For this review, take the finished solid that the model builds, in its own axes (mm). Face numbers are marked on the shaded views. A direction names the side the tool comes from. Round coordinates to 2 decimals unless told otherwise and drop trailing zeros. Order: outer loops, then holes, each group sorted by start corner. A loop starts at its lowest first (then second) coordinate and runs counter-clockwise, first axis right, second up. Notation, with made-up numbers: M 64.5,-39.5 L 92.5,-39.5 A27 cw 92.5,-23.5 Z; hole C -12.75,86 d4. An arc over 180 degrees is marked long. Answer as a JSON object with one key per item and string values.
from build123d import *

# Parameters (mm, degrees)
F0_R     = 19.2
F1_DEPTH = 10
F2_R     = 17
F3_DEPTH = 8
F4_R     = 5.25
F4_R_2   = 3.35
F5_DEPTH = 10
F7_DEPTH = 9
F8_W     = 1
F8_H     = 1
F9_DEPTH = 10


with BuildPart() as f1:
    # F0 (on Top) → F1 (new body)
    with BuildSketch(Plane.XY):
        Circle(F0_R)
    extrude(amount=F1_DEPTH)

    # F2 (on Top) → F3 (cut)
    with BuildSketch(Plane.XY):
        Circle(F2_R)
    extrude(amount=F3_DEPTH, mode=Mode.SUBTRACT)

    # F4 (on Top) → F5 (join)
    with BuildSketch(Plane.XY):
        Circle(F4_R)
        Circle(F4_R_2, mode=Mode.SUBTRACT)
    extrude(amount=F5_DEPTH)

    # F6 (on Top) → F7 (join)
    with BuildSketch(Plane.XY):
        with BuildLine():
            Line((4.017093, -1.060893), (-3.993784, -1.060893))
            ThreePointArc((-3.993784, -1.060893), (0.011655, -3.969964), (4.017093, -1.060893))
        make_face()
    extrude(amount=F7_DEPTH)

    # F8 (on Top) → F9 (join)
    with BuildSketch(Plane.XY):
        with Locations((0, -19.229485)):
            Rectangle(F8_W, F8_H)
    extrude(amount=F9_DEPTH)


solid = f1.part
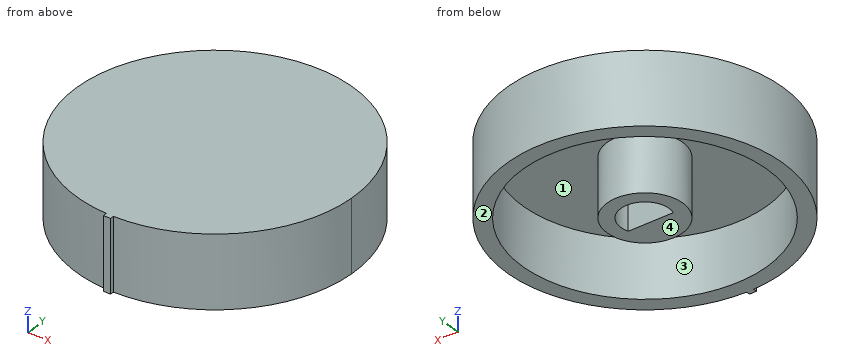
1) For L1, parallel to Y at x = 0, z = 5.25; L2, parallel to X at y = -2, z = 4.5; L3, parallel to X at y = 1, z = 2.5, list the stretches that pass through material, from the lowest coordinate up.
Geometry check:
{"L1": "y = -19.73 to -17, -5.25 to -1.06, 3.35 to 5.25, 17 to 19.2", "L2": "x = -19.1 to -16.88, -4.85 to 4.85, 16.88 to 19.1", "L3": "x = -19.17 to -16.97, -5.15 to -3.2, 3.2 to 5.15, 16.97 to 19.17"}
2) Add section A-A on z = 4.5. State the section outline as (x, y) points.
Geometry check:
{"outline": "C 0,0 d10.5; M -0.5,-19.73 L 0.5,-19.73 L 0.5,-19.19 A19.2 ccw long -0.5,-19.19 Z; hole C 0,0 d34; hole M -3.18,-1.06 L 3.18,-1.06 A3.35 ccw long Z"}
3) Mouldability with a two-part tool opening along X and no side actions: class the marked faces 1 and 2 as +X half, -X half, draft (parallel to the pull), parting line (faces both ways), or undercut.
Geometry check:
{"face 1": "undercut", "face 2": "draft"}
4) Add section B-B on x = 0. State the section outline as (y, z) points, and give its area (3 significant figures).
Geometry check:
{"outline": "M -19.73,0 L -17,0 L -17,8 L -5.25,8 L -5.25,0 L -1.06,0 L -1.06,8 L 3.35,8 L 3.35,0 L 5.25,0 L 5.25,8 L 17,8 L 17,0 L 19.2,0 L 19.2,10 L -19.73,10 Z", "area": "166 mm²"}
5) Insertion check: P1, Ø1.3, axis at x = -1.5, y = 0.5, coming from the -Z side; P2, Ø6, axis at x = 7, z = 5.5, coming from the +Y side; P3, Ø6, axis at y = -8, z = 3.5, coming from the -X side. Each pin has a flat end and moves straight along its axis. Give the tip position at first contact, or say it passes through.
Geometry check:
{"P1": "stops at z = 8", "P2": "stops at y = 18.78", "P3": "stops at x = -18.54"}
6) Machinability: for the marked faces 3 and 4, which of the approach directions +Z, -Z, +X, -X, +Y, -Y give a long, thin tool a straight path to every point of the face, cutting with its end or side? Answer none if there is none.
Geometry check:
{"face 3": "-Z", "face 4": "-Z, +X, -X, +Y, -Y"}
7) Add section C-C on y = 10. State the section outline as (x, z) points.
Geometry check:
{"outline": "M -16.39,0 L -13.75,0 L -13.75,8 L 13.75,8 L 13.75,0 L 16.39,0 L 16.39,10 L -16.39,10 Z"}
8) Add section D-D on z = 8.5. State the section outline as (x, y) points.
Geometry check:
{"outline": "M -0.5,-19.73 L 0.5,-19.73 L 0.5,-19.19 A19.2 ccw long -0.5,-19.19 Z"}
